The listing builds one solid part. Answer for the finished solid, in the listing's coordinates (mm). A direction names the side the tool comes from. Round coordinates to 2 decimals unless told otherwise and drop trailing zeros. Order: outer loops, then holes, each group sorted by start corner. A loop starts at its lowest first (then second) coordinate and runs counter-clockwise, first axis right, second up. Notation, with made-up numbers: (87, -31) -> (104, -31) arc R18 cw to (104, -18) -> close; hole circle Ø7 at (13.5, -4). An arc over 180 degrees is marked (long way). Answer in a Markdown table with one row per item. Add a question column.
```python
from build123d import *

# Parameters (mm, degrees)
SKETCH_1_W          = 50
SKETCH_1_H          = 20
EXTRUDE_1_DEPTH     = 3
SKETCH_2_W          = 50
SKETCH_2_H          = 15
EXTRUDE_2_DEPTH     = 6
SKETCH_5_W          = 50
SKETCH_5_H          = 12
CUT_EXTRUDE_2_DEPTH = 3
SKETCH_6_W          = 10
SKETCH_6_H          = 15
SKETCH_6_R          = 1.65
EXTRUDE_3_DEPTH     = 3
FILLET_1_R          = 1


with BuildPart() as part:
    # 草图1 → 凸台-拉伸1 (new body)
    with BuildSketch(Plane.XY):
        Rectangle(SKETCH_1_W, SKETCH_1_H)
        with BuildLine():
            Line((-4.708438024, 2.5), (4.708438024, 2.5))
            ThreePointArc((4.708438024, 2.5), (5.261208823, 2.666666667), (5.629722688, 3.111111111))
            ThreePointArc((5.629722688, 3.111111111), (21, 0), (5.629722688, -3.111111111))
            ThreePointArc((5.629722688, -3.111111111), (5.261208823, -2.666666667), (4.708438024, -2.5))
            Line((4.708438024, -2.5), (-4.708438024, -2.5))
            ThreePointArc((-4.708438024, -2.5), (-5.261208823, -2.666666667), (-5.629722688, -3.111111111))
            ThreePointArc((-5.629722688, -3.111111111), (-21, 0), (-5.629722688, 3.111111111))
            ThreePointArc((-5.629722688, 3.111111111), (-5.261208823, 2.666666667), (-4.708438024, 2.5))
        make_face(mode=Mode.SUBTRACT)
        with BuildLine():
            Line((3.25, 5.5), (-3.25, 5.5))
            ThreePointArc((-3.25, 5.5), (-5, 7.25), (-3.25, 9))
            Line((-3.25, 9), (3.25, 9))
            ThreePointArc((3.25, 9), (5, 7.25), (3.25, 5.5))
        make_face(mode=Mode.SUBTRACT)
    extrude(amount=EXTRUDE_1_DEPTH)

    # 草图2 → 凸台-拉伸2 (add)
    with BuildSketch(Plane(origin=(0, 10, 0), x_dir=(1, 0, 0), z_dir=(0, 1, 0))):
        with Locations((0, -7.5)):
            Rectangle(SKETCH_2_W, SKETCH_2_H)
    extrude(amount=EXTRUDE_2_DEPTH)

    # 草图5 → 切除-拉伸2 (cut)
    with BuildSketch(Plane.XZ.offset(-10)):
        with Locations((0, 9)):
            Rectangle(SKETCH_5_W, SKETCH_5_H)
    extrude(amount=-CUT_EXTRUDE_2_DEPTH, mode=Mode.SUBTRACT)

    # 草图6 → 凸台-拉伸3 (add)
    # profile 1 of 2: a face of its own
    with BuildSketch(Plane(origin=(0, 16, 0), x_dir=(1, 0, 0), z_dir=(0, 1, 0))):
        with Locations((30, -7.5)):
            Rectangle(SKETCH_6_W, SKETCH_6_H)
        with Locations(Location((30, -7.5, 0), (0, 0, 180))):
            Circle(SKETCH_6_R, mode=Mode.SUBTRACT)
    # profile 2 of 2: a face of its own
    with BuildSketch(Plane(origin=(0, 16, 0), x_dir=(1, 0, 0), z_dir=(0, 1, 0))):
        with Locations((-30, -7.5)):
            Rectangle(SKETCH_6_W, SKETCH_6_H)
        with Locations(Location((-30, -7.5, 0), (0, 0, 180))):
            Circle(SKETCH_6_R, mode=Mode.SUBTRACT)
    extrude(amount=-EXTRUDE_3_DEPTH)

    # 圆角1
    fillet_1_edges = [part.edges().sort_by_distance(p)[0] for p in [
        (25, 13, 1.5),
        (-25, 13, 1.5),
    ]]
    fillet(fillet_1_edges, radius=FILLET_1_R)


solid = part.part
```
1. For faces 5 (the flat face through (0, 15, 15)), 6 (the cylindrical face through (-5, 7.2, 1.5)), 7 (the flat face through (-25, 1, 2)), 8 (the flat face through (25, 1, 2)), determine the directions among +Z, -Z, +X, -X, +Y, -Y from which every point of the face is accessible in a straight line to the end or side of a thin tool.
2. Each of these flat-tipped pins is pushed along its axis until it touches: pin 1 (4.5 mm diameter, centred on x = -15.5, z = 5.5, fed in from -Y); pin 2 (2.5 mm diameter, centred on y = -3, z = 1.5, fed in from +X); pin 3 (4 mm diameter, centred on x = 11, y = 7.5, fed in from -Z); pin 4 (1.5 mm diameter, centred on y = 4.5, z = 1.5, fed in from -X). Where does it stop, or does it pass through?
3. The part is cut by section B-B (z = 7.5). Give the vertices of the cut face in (x, y).
4. The part is cut by section D-D (x = 0.5). Give the vertices of the cut face in (y, z).
5. The part is cut by section A-A (x = -13). Give the vertices of the cut face in (y, z).
6. The mould has two halves that part along Z. Classify faces 1 (the flat face through (0, 3, 0)), 2 (the cylindrical face through (-28.35, 14.52, 7.57)), 3 (the flat face through (0, -2.5, 1)), 4 (the flat face through (0, 4, 3)): released by +Z, released by -Z, zero draft, split by the parting line, or undercut.
7. The part is cut by section C-C (y = 0). Give the vertices of the cut face in (x, z), then the cut area to 3 significant figures.
8. Straight lines are drawn through the part: line 1 along Z through (x, y) = (-30, 14.35); line 2 along Y through (x, z) = (-13, 1); line 3 along Y through (x, z) = (30.5, 10.5). For each, find the intervals that lie inside material, in ascending order.
Report:
| question | item | result |
|---|---|---|
| 1 | face 5 | +Z, +X, -X, +Y, -Y |
| 1 | face 6 | +Z, -Z |
| 1 | face 7 | +Z, -Z, -X, -Y |
| 1 | face 8 | +Z, -Z, +X, -Y |
| 2 | pin 1 | stops at y = 13 |
| 2 | pin 2 | stops at x = 25 |
| 2 | pin 3 | stops at z = 0 |
| 2 | pin 4 | stops at x = -25 |
| 3 | outline | (-35, 13) -> (-31.65, 13) -> (-31.65, 16) -> (-35, 16) -> close; (-28.35, 13) -> (28.35, 13) -> (28.35, 16) -> (-28.35, 16) -> close; (31.65, 13) -> (35, 13) -> (35, 16) -> (31.65, 16) -> close |
| 4 | outline | (-10, 0) -> (-2.5, 0) -> (-2.5, 3) -> (-10, 3) -> close; (2.5, 0) -> (5.5, 0) -> (5.5, 3) -> (2.5, 3) -> close; (9, 0) -> (16, 0) -> (16, 15) -> (13, 15) -> (13, 3) -> (9, 3) -> close |
| 5 | outline | (-10, 0) -> (-8, 0) -> (-8, 3) -> (-10, 3) -> close; (8, 0) -> (16, 0) -> (16, 15) -> (13, 15) -> (13, 3) -> (8, 3) -> close |
| 6 | face 1 | released by -Z |
| 6 | face 2 | undercut |
| 6 | face 3 | zero draft |
| 6 | face 4 | released by +Z |
| 7 | outline | (-25, 0) -> (-21, 0) -> (-21, 3) -> (-25, 3) -> close; (21, 0) -> (25, 0) -> (25, 3) -> (21, 3) -> close |
| 7 | area | 24.0 mm^2 |
| 8 | line 1 | z = 0 to 5.85, 9.15 to 15 |
| 8 | line 2 | y = -10 to -8, 8 to 16 |
| 8 | line 3 | y = 13 to 16 |
